```python
from build123d import *

# Parameters (mm, degrees)
SKETCH1_R           = 90
BOSS_EXTRUDE1_DEPTH = 5
SKETCH2_W           = 15
SKETCH2_H           = 35
BOSS_EXTRUDE2_DEPTH = 110
CUT_EXTRUDE1_DEPTH  = 36
SKETCH4_R           = 2.18255
CUT_EXTRUDE2_DEPTH  = 62


with BuildPart() as part:
    # Sketch1 → Boss-Extrude1 (new body)
    with BuildSketch(Plane(origin=(0, 0, 0), x_dir=(1, 0, 0), z_dir=(0, 1, 0))):
        with Locations(Location((0, 0, 0), (0, 0, 270))):
            Circle(SKETCH1_R)
    extrude(amount=BOSS_EXTRUDE1_DEPTH)

    # Sketch2 → Boss-Extrude2 (add)
    with BuildSketch(Plane(origin=(0, 5, 0), x_dir=(1, 0, 0), z_dir=(0, 1, 0))):
        Rectangle(SKETCH2_W, SKETCH2_H)
    extrude(amount=BOSS_EXTRUDE2_DEPTH)

    # Sketch3 → Cut-Extrude1 (cut)
    with BuildSketch(Plane.XY.offset(17.5)):
        Polygon((-2.373551685, 115), (2.826448315, 115), (5.726448315, 109.977052658), (-5.273551685, 109.977052658), align=None)
    extrude(amount=-CUT_EXTRUDE1_DEPTH, mode=Mode.SUBTRACT)

    # Sketch4 → Cut-Extrude2 (cut)
    with BuildSketch(Plane(origin=(0, 0, 0), x_dir=(-1, 0, 0), z_dir=(0, -1, 0))):
        with Locations(Location((-26.585, 79.907325251, 0), (0, 0, 90))):
            Circle(SKETCH4_R)
        with Locations(Location((26.585, 79.907325251, 0), (0, 0, 90))):
            Circle(SKETCH4_R)
        with Locations(Location((82.310329065, -16.825152102, 0), (0, 0, 90))):
            Circle(SKETCH4_R)
        with Locations(Location((56.093218167, -63.082173149, 0), (0, 0, 90))):
            Circle(SKETCH4_R)
        with Locations(Location((26.585, -79.907325251, 0), (0, 0, 90))):
            Circle(SKETCH4_R)
        with Locations(Location((-26.585, -79.907325251, 0), (0, 0, 90))):
            Circle(SKETCH4_R)
        with Locations(Location((-53.346563788, -64.612502947, 0), (0, 0, 90))):
            Circle(SKETCH4_R)
        with Locations(Location((-82.245302282, -19.978089739, 0), (0, 0, 90))):
            Circle(SKETCH4_R)
    extrude(amount=-CUT_EXTRUDE2_DEPTH, mode=Mode.SUBTRACT)


solid = part.part
```
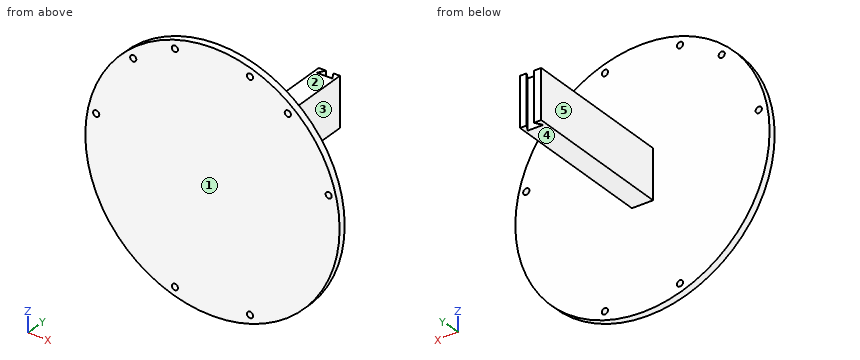
Verification items for the finished model (mm, model axes). Face numbers are marked on the shaded views. A direction names the side the tool comes from. Give positions to 0.01 mm unless a question says otherwise; leave off trailing zeros. Order: outer loops, then holes, each group sorted by start corner. A loop starts at its lowest first (then second) coordinate and runs counter-clockwise, first axis right, second up. Notation, with made-up numbers: M 36,-18.75 L 47,-18.75 A25 ccw 47,13.25 Z; hole C 86.25,74.25 d5. An arc over 180 degrees is marked long. Answer in a Markdown table with one row per item. Add a question column.
Item 1: Tool access check on the marked faces 1, 2, 3, 4 and 5. Record the directions out of +Z, -Z, +X, -X, +Y, -Y that give a thin tool (end or side, any length) a straight path to the whole face; none if there is none.
Item 2: Section check A-A, the plane z = 0. Enter the section's corners in (x, y).
Item 3: Section check D-D, the plane z = -46. Enter the section's corners in (x, y), and give its area (3 significant figures).
Item 4: Section check B-B, the plane x = 0. Enter the section's corners in (y, z).
Item 5: Section check C-C, the plane y = 14. Enter the section's corners in (x, z), and give its area (3 significant figures).
Item 6: Gauge pin test, flat ends, axial feed: pin 1 (2 mm diameter, centred on y = 41, z = -11.5, fed in from +X); pin 2 (2 mm diameter, centred on x = -14, z = -65, fed in from +Y); pin 3 (16.5 mm diameter, centred on x = -1.5, y = 34.5, fed in from +Z). Record the tip position at first contact, or that the pin passes through.
Item 7: Scan lines: probe 1 along Y at (x, z) = (-80, -11.5); probe 2 along X at (y, z) = (53, 13.5); probe 3 along Z at (x, y) = (-5.5, 106). Record each from-to range of solid material in increasing order. Write a range as from..to.
Filled sheet:
| question | item | result |
|---|---|---|
| 1 | face 1 | +Z, -Z, +X, -X, -Y |
| 1 | face 2 | +Z, +X, -X, +Y |
| 1 | face 3 | +Z, -Z, +X, +Y |
| 1 | face 4 | -Z, +X, -X, +Y |
| 1 | face 5 | +Z, -Z, -X, +Y |
| 2 | outline | M -90,0 L 90,0 L 90,5 L 7.5,5 L 7.5,115 L 2.83,115 L 5.73,109.98 L -5.27,109.98 L -2.37,115 L -7.5,115 L -7.5,5 L -90,5 Z |
| 3 | outline | M -77.36,0 L 77.36,0 L 77.36,5 L -77.36,5 Z |
| 3 | area | 774 mm^2 |
| 4 | outline | M 0,-90 L 5,-90 L 5,-17.5 L 109.98,-17.5 L 109.98,17.5 L 5,17.5 L 5,90 L 0,90 Z |
| 5 | outline | M -7.5,-17.5 L 7.5,-17.5 L 7.5,17.5 L -7.5,17.5 Z |
| 5 | area | 525 mm^2 |
| 6 | pin 1 | stops at x = 7.5 |
| 6 | pin 2 | stops at y = 5 |
| 6 | pin 3 | stops at z = 17.5 |
| 7 | probe 1 | y = 0..5 |
| 7 | probe 2 | x = -7.5..7.5 |
| 7 | probe 3 | z = -17.5..17.5 |
